Can you work these out from the model? Positions are in its coordinate system, mm. A direction names the side the tool comes from. Give positions to 0.01 mm unless a question says otherwise; leave off trailing zeros. Loops run counter-clockwise (first coordinate to the right, second up) from the corner with the lowest first, then second, coordinate; pieces in that order, holes last. Notation, with made-up numbers: (45, 60.5) -> (76, 60.5) arc R12 cw to (76, 68.5) -> close; hole circle Ø8 at (46, 84). An arc over 180 degrees is marked (long way). One line per question, with ' | ' between items.
from build123d import *

# Parameters (mm, degrees)
SKETCH1_W           = 20
SKETCH1_H           = 2.5
BOSS_EXTRUDE1_DEPTH = 30
SKETCH2_W           = 40
SKETCH2_H           = 40
BOSS_EXTRUDE2_DEPTH = 20
FILLET1_R           = 10


with BuildPart() as part:
    # Sketch1 → Boss-Extrude1 (new body)
    with BuildSketch(Plane.XY):
        with Locations((-20, -1.25)):
            Rectangle(SKETCH1_W, SKETCH1_H)
    extrude(amount=BOSS_EXTRUDE1_DEPTH)

    # Sketch2 → Boss-Extrude2 (add)
    with BuildSketch(Plane.XY):
        with Locations((-10, 17.5)):
            Rectangle(SKETCH2_W, SKETCH2_H)
    extrude(amount=-BOSS_EXTRUDE2_DEPTH)

    # Fillet1
    # the kernel refuses this fillet: 10 mm, written as the material it adds along each edge
    with BuildSketch(Plane(origin=(-10, 0, 0), x_dir=(0, 1, 0), z_dir=(-1, 0, 0))) as fillet1_piece_1:
        with BuildLine():
            CenterArc((FILLET1_R, -FILLET1_R), FILLET1_R, 90, 90)
            Line((0, -FILLET1_R), (0, 0))
            Line((0, 0), (FILLET1_R, 0))
        make_face()
    extrude(amount=20)
    # the kernel refuses this fillet: 10 mm, written as the material it takes off along each edge
    with BuildSketch(Plane(origin=(10, 37.5, 25), x_dir=(-1, 0, 0), z_dir=(0, 0, -1))) as fillet1_2_piece_1:
        with BuildLine():
            CenterArc((FILLET1_R, -FILLET1_R), FILLET1_R, 90, 90)
            Line((0, -FILLET1_R), (0, 0))
            Line((0, 0), (FILLET1_R, 0))
        make_face()
    extrude(amount=70, mode=Mode.SUBTRACT)
    with BuildSketch(Plane(origin=(6.535945694, 0, 30), x_dir=(0, 0, -1), z_dir=(-1, 0, 0))) as fillet1_2_piece_2:
        with BuildLine():
            CenterArc((6.614378278, 10), FILLET1_R, 228.590377891, 41.409622109)
            Line((0, 2.5), (0, 0))
            Line((0, 0), (6.614378278, 0))
        make_face()
    extrude(amount=53.071891388, mode=Mode.SUBTRACT)


solid = part.part
Q1. If we section it at C-C (y = 1): Write out the boundary of the cut face in (x, z).
Entries:
outline: (-30, -20) -> (10, -20) -> (10, 0) -> (-10, 0) -> (-10, 5.64) -> (-30, 5.64) -> close
Q2. On a 3-axis mill with a long thin cutter (end or side, diameter ignored), from which of +Z, -Z, +X, -X, +Y, -Y can I reach the whole of each face in a straight line? I mean faces 1 (the face through (-10, -0.4, 11.6)), 2 (the face through (-10, 22, 0)), 3 (the face through (-20, 0, 17)). Say none if no direction works.
Entries:
face 1: +Z, +X, +Y, -Y | face 2: +Z, +X, +Y | face 3: +Z, +X, -X, +Y
Q3. If we section it at A-A (x = -14): Write out the boundary of the cut face in (y, z), plus the area to 3 significant figures.
Entries:
outline: (-2.5, -20) -> (37.5, -20) -> (37.5, 0) -> (10, 0) arc R10 cw to (0, 10) -> (0, 23.39) arc R10 ccw to (-2.5, 30) -> close | area: 891 mm²
Q4. If I drill on probe 1 along Z at (x, y) = (-1.5, 12); probe 2 along X at (y, z) = (28, -4.5); probe 3 along Y at (x, z) = (-17.5, 20), over which ranges is the centre line in solid material (lowest first)? Write a range as from..to.
Entries:
probe 1: -20..0 | probe 2: -30..9.99 | probe 3: -2.5..0
Q5. If we section it at D-D (x = -7.5): Write out the boundary of the cut face in (y, z).
Entries:
outline: (-2.5, -20) -> (37.5, -20) -> (37.5, 0) -> (-2.5, 0) -> close
Q6. If we section it at B-B (z = 21): Write out the boundary of the cut face in (x, y).
Entries:
outline: (-30, -2.5) -> (-10, -2.5) -> (-10, 0) -> (-30, 0) -> close
Q7. For pin 1 Ø6 at (y, z) = (18, 0.5) entering from +X; pin 2 Ø10 at (x, y) = (-20.5, 27.5) entering from +Z; pin 3 Ø14.5 at (x, z) = (-21.5, 14.5) entering from +Y; pin 4 Ø1.5 at (x, z) = (-9.5, 17.5) entering from +Y, each with a flat end and sliding along its axis, tell me the tip position at first contact or that it passes through.
Entries:
pin 1: x = 10 | pin 2: z = 0 | pin 3: y = 0.39 | pin 4: y = 0
